Autodesk Inventor part; units mm, degrees
ref_plane "YZ Plane" through (0, 0, 0) normal (1, 0, 0) x (0, 1, 0)
ref_plane "XZ Plane" through (0, 0, 0) normal (0, 1, 0) x (-1, 0, 0)
ref_plane "XY Plane" through (0, 0, 0) normal (0, 0, 1) x (1, 0, 0)
sketch "草圖1" plane through (0, 0, 0) normal (0, 1, 0) x (-1, 0, 0)
  line L0 (29.5719, -39.0966) -> (29.5719, -13.0966)
  line L1 (29.5719, -39.0966) -> (-0.4281, -39.0966)
  point P0 (0, 0)
  dimension "d0" = 26
  dimension "d2" = 90
  dimension "d3" = 30
contour flange "輪廓線凸緣1" sketch "草圖1" thickness 0.5 bend radius 0.5 width 25 along (0, 1, 0) mid plane no both sides no wall seen from (-29.5719, 0, -26.0966) lies toward (1, 0, 0) curves L0 L1
bend "折彎1"
corner "轉角1"
sketch "草圖2" plane through (-29.0719, 0, -13.0966) normal (1, 0, 0) x (0, 0, -1)
  circle A0 centre (12.5, 12.5) radius 12.5
  line L0 (0, 25) -> (25, 25)
  line L1 (0, 0) -> (0, 25)
  line L2 (0, 0) -> (25, 0)
  point P0 (-13.0966, 0)
  point P1 (0, 12.5)
  point P2 (12.5, 25)
  point P3 (12.5, 0)
  dimension "d15" = 25
extrude "擠出1" cut sketch "草圖2" against normal up to surface (0.5 mm away) contours A0 L1 L0 | L2 L1 A0
sketch "草圖3" plane through (-29.0719, 0, -38.0966) normal (1, 0, 0) x (0, 0, -1)
  arc A0 (-12.5, 25) -> (-12.5, 0) centre (-12.5, 12.5) ccw
  circle A1 centre (-12.5, 21) radius 1.5
  circle A2 centre (-12.5, 4) radius 1.5
  point P0 (-38.0966, 0)
  dimension "d18" = 3
  dimension "d19" = 17
  dimension "d20" = 8.5
  dimension "d21" = 3
extrude "擠出2" cut sketch "草圖3" against normal up to surface (0.5 mm away)
sketch "草圖4" plane through (0.4281, 0, -38.5966) normal (0, 0, 1) x (1, 0, 0)
  circle A0 centre (-23, 21) radius 1.5
  circle A1 centre (-3, 21) radius 1.5
  circle A2 centre (-23, 4) radius 1.5
  circle A3 centre (-3, 4) radius 1.5
  line L0 (0, 0) -> (0, 25)
  line L1 (-3, 21) -> (-3, 4)
  line L2 (-3, 12.5) -> (-13.1347, 12.5)
  line L3 (-29, 25) -> (0, 25)
  point P0 (-0.4281, 0)
  dimension "d24" = 20
  dimension "d25" = 3
  dimension "d26" = 3
  dimension "d27" = 3
  dimension "d28" = 3
  dimension "d29" = 17
  dimension "d30" = 3
  dimension "d31" = 12.5
extrude "擠出3" cut sketch "草圖4" against normal up to surface (0.5 mm away)
sketch "草圖5" plane through (-29.0719, 0, -38.0966) normal (1, 0, 0) x (0, 0, -1)
  arc A0 (-12.5, 25) -> (-12.5, 0) centre (-12.5, 12.5) ccw
  circle A1 centre (-12.5, 12.5) radius 3.5
  point P0 (-38.0966, 0)
  dimension "d34" = 7
extrude "擠出4" cut sketch "草圖5" against normal up to surface (0.5 mm away)
equation "\"d4\" = 厚度"
equation "\"d5\" = 折彎離隙寬度"
equation "\"d6\" = 折彎離隙深度"
equation "\"d7\" = 最小剩餘"
equation "\"d8\" = 轉移半徑"
equation "\"d10\" = 折彎半徑"
equation "\"d12\" = 轉角離隙大小"
equation "\"d13\" = 間隙大小"
equation "\"d14\" = Jacobi半徑大小"
equation "\"折彎半徑\" = 厚度"
equation "\"折彎離隙寬度\" = 厚度"
equation "\"折彎離隙深度\" = 0.5 * 厚度"
equation "\"轉角離隙大小\" = 4 * 厚度"
equation "\"最小剩餘\" = 2 * 厚度"
equation "\"轉移半徑\" = 折彎半徑"
equation "\"Jacobi半徑大小\" = 折彎半徑"
equation "\"間隙大小\" = 厚度"
properties part number "motor_base"
Verification items for the finished model (mm, model axes). A direction names the side the tool comes from. Give positions to 0.01 mm unless a question says otherwise; leave off trailing zeros. Order: outer loops, then holes, each group sorted by start corner. A loop starts at its lowest first (then second) coordinate and runs counter-clockwise, first axis right, second up. Notation, with made-up numbers: M 52.25,75.5 L 56.25,75.5 A21 ccw 56.25,104.5 Z; hole C 46,75.5 d5. An arc over 180 degrees is marked long. Return JSON: item names as keys, results as strings. Group by question number.
1) Go/stop test with flat-tipped pins: pin 1 Ø1.8 at (y, z) = (4, -25.6) entering from +X (3 decimals); pin 2 Ø3.5 at (y, z) = (21, -25.6) entering from +X; pin 3 Ø5 at (x, y) = (-3.5, 7) entering from +Z. Record where each tip stops, or that it passes through.
2) Scan lines: line 1 (Z direction, x = -25.5, y = 13.5); line 2 (X direction, y = 19.5, z = -20.5). Record each from-to range of solid material in increasing order.
3) Access from +Z, -Z, +X, -X, +Y, -Y to the whole of each face (thin tool, end or side, straight path). Record for faces 4 (the face through (-29.072, 15, -29)), 5 (the face through (-21.14, 4.45, -38.84)).
4) Section check B-B on y = 20.25. Record the cut outline in (x, z).
5) Section check A-A on y = 12.5. Record the cut outline in (x, z), and give its area (3 significant figures).
6) Mould release check, pull along Y, two halves, no side actions. Record for faces 1 (the face through (-29.318, 21.451, -27.027)), 2 (the face through (-14, 12, -38.597)), 3 (the face through (-29.3, 12.8, -13.1)): pulls with the +Y half, pulls with the -Y half, needs draft (parallel to the pull), parting line crosses it, or undercut.
7) Section check D-D on y = 4.5. Record the cut outline in (x, z).
8) Section check C-C on x = -5.25. Record the cut outline in (y, z).
Answer block:
{
 "1": {"pin 1": "passes through", "pin 2": "stops at x = -29.07", "pin 3": "stops at z = -38.6"},
 "2": {"line 1": "z = -39.1 to -38.6", "line 2": "x = -29.57 to -29.07"},
 "3": {"face 4": "+Z, +X, +Y, -Y", "face 5": "+Z, -Z"},
 "4": {"outline": "M -29.57,-38.1 A1 ccw -28.57,-39.1 L -23.87,-39.1 L -23.87,-38.6 L -28.57,-38.6 A0.5 cw -29.07,-38.1 L -29.07,-26.9 L -29.57,-26.9 Z; M -29.57,-24.3 L -29.07,-24.3 L -29.07,-15.79 L -29.57,-15.79 Z; M -21.27,-39.1 L -3.87,-39.1 L -3.87,-38.6 L -21.27,-38.6 Z; M -1.27,-39.1 L 0.43,-39.1 L 0.43,-38.6 L -1.27,-38.6 Z"},
 "5": {"outline": "M -29.57,-38.1 A1 ccw -28.57,-39.1 L 0.43,-39.1 L 0.43,-38.6 L -28.57,-38.6 A0.5 cw -29.07,-38.1 L -29.07,-29.1 L -29.57,-29.1 Z; M -29.57,-22.1 L -29.07,-22.1 L -29.07,-13.1 L -29.57,-13.1 Z", "area": "24.1 mm^2"},
 "6": {"face 1": "undercut", "face 2": "needs draft", "face 3": "parting line crosses it"},
 "7": {"outline": "M -29.57,-38.1 A1 ccw -28.57,-39.1 L -23.99,-39.1 L -23.99,-38.6 L -28.57,-38.6 A0.5 cw -29.07,-38.1 L -29.07,-27.01 L -29.57,-27.01 Z; M -29.57,-24.18 L -29.07,-24.18 L -29.07,-15.99 L -29.57,-15.99 Z; M -21.16,-39.1 L -3.99,-39.1 L -3.99,-38.6 L -21.16,-38.6 Z; M -1.16,-39.1 L 0.43,-39.1 L 0.43,-38.6 L -1.16,-38.6 Z"},
 "8": {"outline": "M 0,-39.1 L 25,-39.1 L 25,-38.6 L 0,-38.6 Z"}
}
